Source: CAD feature listing. Evaluate the final solid. Frame: model axes, mm. A direction names the side the tool comes from. Give positions to 0.01 mm unless a question says otherwise; leave off trailing zeros. Loops run counter-clockwise (first coordinate to the right, second up) from the corner with the lowest first, then second, coordinate; pieces in that order, holes last. Notation, with made-up numbers: (41, 42) -> (85, 42) arc R16 cw to (85, 66) -> close; hole circle Ø7 at (82, -12). An arc over 180 degrees is marked (long way). Put each result on its own line as item: value.
```python
from build123d import *

# Parameters (mm, degrees)
F0_W      = 1200
F0_H      = 900
F1_DEPTH  = 40
F2_T      = -1.5
F3_W      = 40
F3_H      = 40
F4_DEPTH  = 818.5
F5_W      = 817
F5_H      = 40
F6_DEPTH  = 40
F7_W      = 817
F7_H      = 40
F8_DEPTH  = 40
F9_W      = 1117
F9_H      = 40
F10_DEPTH = 40


with BuildPart() as f1:
    # F0 (on Top) → F1 (new body)
    with BuildSketch(Plane.XY):
        Rectangle(F0_W, F0_H)
    extrude(amount=F1_DEPTH)

    # F2
    f2_openings = [f1.faces().sort_by_distance(p)[0] for p in [
        (0, 0, 0),
    ]]
    offset(amount=F2_T, openings=f2_openings)

    # F3 (on face) → F4 (join)
    with BuildSketch(Plane(origin=(0, 0, 38.5), x_dir=(1, 0, 0), z_dir=(0, 0, -1))):
        with Locations((-578.5, 428.5)):
            Rectangle(F3_W, F3_H)
        with Locations((578.5, 428.5)):
            Rectangle(F3_W, F3_H)
        with Locations((578.5, -428.5)):
            Rectangle(F3_W, F3_H)
        with Locations((-578.5, -428.5)):
            Rectangle(F3_W, F3_H)
    extrude(amount=F4_DEPTH)

    # F5 (on face) → F6 (join)
    with BuildSketch(Plane(origin=(-598.5, 0, 0), x_dir=(0, -1, 0), z_dir=(-1, 0, 0))):
        with Locations((0, -560)):
            Rectangle(F5_W, F5_H)
    extrude(amount=-F6_DEPTH)

    # F7 (on face) → F8 (join)
    with BuildSketch(Plane(origin=(558.5, 0, 0), x_dir=(0, -1, 0), z_dir=(-1, 0, 0))):
        with Locations((0, -560)):
            Rectangle(F7_W, F7_H)
    extrude(amount=-F8_DEPTH)

    # F9 (on face) → F10 (join)
    with BuildSketch(Plane(origin=(0, 0, -580), x_dir=(1, 0, 0), z_dir=(0, 0, -1))):
        Rectangle(F9_W, F9_H)
    extrude(amount=-F10_DEPTH)


solid = f1.part
```
(1) Draft query along X for faces 1 (the flat face through (-598.5, 2, -562)), 2 (the flat face through (578, 428, -780)), 3 (the flat face through (558.5, 410, -399)). Return one class per face: released by +X, released by -X, zero draft, split by the parting line, or undercut.
Calculated:
face 1: released by -X
face 2: zero draft
face 3: undercut
(2) Section C-C on y = -344.5. Return loops of the section in (x, z).
Calculated:
outline: (-600, 0) -> (-598.5, 0) -> (-598.5, 38.5) -> (598.5, 38.5) -> (598.5, 0) -> (600, 0) -> (600, 40) -> (-600, 40) -> close; (-598.5, -580) -> (-558.5, -580) -> (-558.5, -540) -> (-598.5, -540) -> close; (558.5, -580) -> (598.5, -580) -> (598.5, -540) -> (558.5, -540) -> close
(3) Section A-A on x = -329. Return loops of the section in (y, z), then the cut area to 3 significant figures.
Calculated:
outline: (-450, 0) -> (-448.5, 0) -> (-448.5, 38.5) -> (448.5, 38.5) -> (448.5, 0) -> (450, 0) -> (450, 40) -> (-450, 40) -> close; (-20, -580) -> (20, -580) -> (20, -540) -> (-20, -540) -> close
area: 3,070 mm²
(4) Section B-B on z = -253.5. Return loops of the section in (x, y), then the cut area to 3 significant figures.
Calculated:
outline: (-598.5, -448.5) -> (-558.5, -448.5) -> (-558.5, -408.5) -> (-598.5, -408.5) -> close; (-598.5, 408.5) -> (-558.5, 408.5) -> (-558.5, 448.5) -> (-598.5, 448.5) -> close; (558.5, -448.5) -> (598.5, -448.5) -> (598.5, -408.5) -> (558.5, -408.5) -> close; (558.5, 408.5) -> (598.5, 408.5) -> (598.5, 448.5) -> (558.5, 448.5) -> close
area: 6,400 mm²
(5) Line query: probe 1 along Z at (x, y) = (-417, 397.5). Output: solid intervals per line, ascending. Write a range as from..to.
Calculated:
probe 1: z = 38.5..40
(6) First-contact query: P1, Ø12, axis at x = -583, z = -340.5, coming from the +Y side; P2, Ø12, axis at x = -570, z = -719.5, coming from the -Y side; P3, Ø10, axis at x = 21, y = 207.5, coming from the -Z side. Flat tips, straight axial feed; report the tip coordinate or a pass-through.
Calculated:
P1: stops at y = 448.5
P2: stops at y = -448.5
P3: stops at z = 38.5
(7) Reachability of faces 4 (the flat face through (-579, 448.5, -385)), 5 (the flat face through (-8, 448.5, 19)), 6 (the flat face through (-579, -448.5, -385)), 7 (the flat face through (-3, 2, -580)), 8 (the flat face through (598.5, -6, 19)) from +Z, -Z, +X, -X, +Y, -Y: full face, straight path, thin tool, end or side. Return the list, or none.
Calculated:
face 4: -Z, +X, -X, +Y
face 5: -Z
face 6: -Z, +X, -X, -Y
face 7: -Z, +X, -X
face 8: none
